Design review of the part shown in the three views and the two pictorial views. Dimensions are in mm from the part's minimum x, y and z. A direction names the side the tool comes from. Round coordinates to 2 decimals unless told otherwise and drop trailing zeros. Loops run counter-clockwise (first coordinate to the right, second up) from the corner with the lowest first, then second, coordinate; pieces in that order, holes last. Notation, with made-up numbers: M -2,32 L 48,32 A16 ccw 48,60 Z; hole C -31,39 d10. An arc over 180 degrees is marked long. Answer in a Markdown table with one row per item. Add a question column.
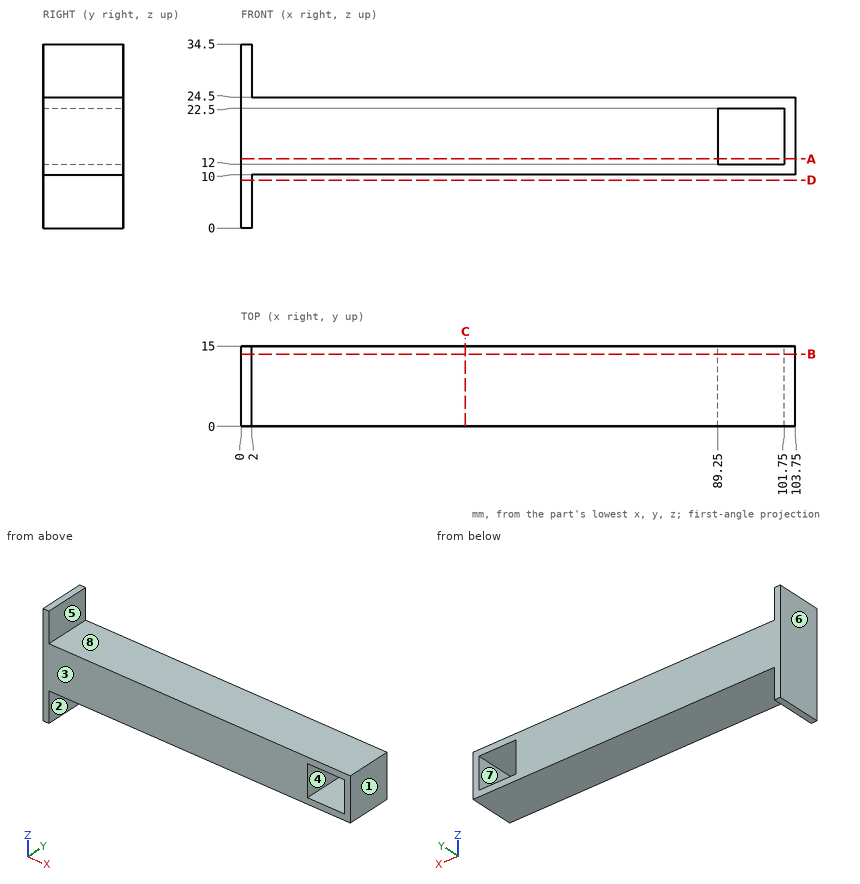
1. For pin 1 Ø8 at (y, z) = (6, 31) entering from +X; pin 2 Ø3 at (y, z) = (7.5, 18.5) entering from -X; pin 3 Ø6 at (x, y) = (97.5, 5) entering from -Z, all flat-tipped, find the tip position at first contact; note any pin that passes through.
2. Take a section at B-B, the plane y = 13.5. State the section outline as (x, z) points.
3. Mouldability with a two-part tool opening along X and no side actions: class the marked faces 6, 7 and 8 as released by +X, released by -X, zero draft, split by the parting line, or undercut.
4. To check wall thickness, follow probe 1 along X at (y, z) = (4, 19); probe 2 along Z at (x, y) = (96.5, 7.25); probe 3 along Z at (x, y) = (70, 9). State the ranges of each line that lie inside material, in increasing order.
5. Take a section at C-C, the plane x = 42. State the section outline as (y, z) points, and give its area (4 significant figures).
6. Take a section at D-D, the plane z = 9. State the section outline as (x, y) points, and give its area (3 significant figures).
7. Take a section at A-A, the plane z = 13. State the section outline as (x, y) points, and give its area (3 significant figures).
8. Machinability: for the marked faces 1, 2, 3, 4 and 5, which of the approach directions +Z, -Z, +X, -X, +Y, -Y give a long, thin tool a straight path to every point of the face, cutting with its end or side? Answer none if there is none.
Check sheet entries:
| question | item | result |
|---|---|---|
| 1 | pin 1 | stops at x = 2 |
| 1 | pin 2 | stops at x = 0 |
| 1 | pin 3 | stops at z = 10 |
| 2 | outline | M 0,0 L 2,0 L 2,10 L 103.75,10 L 103.75,24.5 L 2,24.5 L 2,34.5 L 0,34.5 Z; hole M 89.25,12 L 101.75,12 L 101.75,22.5 L 89.25,22.5 Z |
| 3 | face 6 | released by -X |
| 3 | face 7 | undercut |
| 3 | face 8 | zero draft |
| 4 | probe 1 | x = 0 to 89.25, 101.75 to 103.75 |
| 4 | probe 2 | z = 10 to 12, 22.5 to 24.5 |
| 4 | probe 3 | z = 10 to 24.5 |
| 5 | outline | M 0,10 L 15,10 L 15,24.5 L 0,24.5 Z |
| 5 | area | 217.5 mm^2 |
| 6 | outline | M 0,0 L 2,0 L 2,15 L 0,15 Z |
| 6 | area | 30.0 mm^2 |
| 7 | outline | M 0,0 L 89.25,0 L 89.25,15 L 0,15 Z; M 101.75,0 L 103.75,0 L 103.75,15 L 101.75,15 Z |
| 7 | area | 1,370 mm^2 |
| 8 | face 1 | +Z, -Z, +X, +Y, -Y |
| 8 | face 2 | -Z, +X, +Y, -Y |
| 8 | face 3 | +Z, -Z, +X, -X, -Y |
| 8 | face 4 | +Y, -Y |
| 8 | face 5 | +Z, +X, +Y, -Y |
